Check sheet for the modelled part. Datum: model origin and axes. Units: mm. A direction names the side the tool comes from. Round coordinates to 2 decimals unless told otherwise and drop trailing zeros. Write each loop counter-clockwise with the first axis right and the second up, starting at its lowest first coordinate (ties: lowest second). Pieces come first, ordered by that corner, then holes.
Item 1: Section check A-A, the plane y = -14.5. Record the cut outline in (x, z).
Item 2: Depth check by flat-ended pin: pin 1 (18 mm diameter, centred on y = -20, z = -52.29, fed in from -X); pin 2 (10 mm diameter, centred on y = -25, z = 103, fed in from -X); pin 3 (3 mm diameter, centred on y = -24.5, z = -48.5, fed in from +X). Enter the tip coordinate at first touch or a pass-through.
Item 3: Section check D-D, the plane x = -81. Record the cut outline in (y, z), plus the area to 3 significant figures.
Item 4: Set-up check for faces 1 (the cylindrical face through (73.36, -24.22, -71.32)), 2 (the flat face through (-1, -20, -32.294)), 3 (the flat face through (-12.548, -19.789, 98.794)), 4 (the flat face through (-60, 0, -21)): record each of +Z, -Z, +X, -X, +Y, -Y from which the full face is reachable in a straight line by a thin tool's end or side.
Item 5: Section check C-C, the plane z = -24. Record the cut outline in (x, y).
Item 6: Material ranges on line 1 along Z through (x, y) = (73.5, -20); line 2 along Y through (x, z) = (74, -51); line 3 along Z through (x, y) = (55, -7), recorded low to high.
Item 7: Release check for a two-part mould opening along Z. For faces 5 (the flat face through (86.036, -10, -64)), 6 (the flat face through (-13.932, -0.647, 99.594)), 7 (the flat face through (-38, -20, -72.294)) record: pulls with the +Z half, pulls with the -Z half, needs draft (parallel to the pull), parting line crosses it, or undercut.
Item 8: Section check B-B, the plane x = -21. State how many separate pieces and enclosed holes the cut face has, plus the area to 3 significant figures.
from build123d import *

# Parameters (mm, degrees)
F1_DEPTH = 40
F2_R     = 19.0977324209
F2_R_2   = 15.0689951662
F3_DEPTH = 25
F4_R     = 19.4897068619
F4_R_2   = 15.068995
F5_DEPTH = 25


with BuildPart() as f1:
    # F0 (on Front) → F1 (new body)
    with BuildSketch(Plane.XZ):
        Polygon((61.0357465344, -32.2937653869), (-65.3808493135, -32.2937653869), (4.5902623163, 88.899755018), (-30.0507538351, 108.899755018), (-134.6628816163, -72.2937653869), (61.0357465344, -72.2937653869), align=None)
    extrude(amount=F1_DEPTH)

    # F2 (on face) → F3 (join)
    with BuildSketch(Plane(origin=(39.642288697, 0, 68.6624581515), x_dir=(0.8660254038, 0, -0.5), z_dir=(0.5, 0, 0.8660254038))):
        with Locations((-60.4745937331, -20)):
            Circle(F2_R)
        with Locations((-60.4745937331, -20)):
            Circle(F2_R_2, mode=Mode.SUBTRACT)
    extrude(amount=F3_DEPTH)

    # F4 (on face) → F5 (join)
    with BuildSketch(Plane.YZ.offset(61.0357465344)):
        with Locations((-20, -52.2937653869)):
            Circle(F4_R)
        with Locations((-20, -52.2937653869)):
            Circle(F4_R_2, mode=Mode.SUBTRACT)
    extrude(amount=F5_DEPTH)


solid = f1.part
Values found:
1. outline: (-134.66, -72.29) - (61.04, -72.29) - (61.04, -70.99) - (86.04, -70.99) - (86.04, -66.32) - (61.04, -66.32) - (61.04, -38.26) - (86.04, -38.26) - (86.04, -33.6) - (61.04, -33.6) - (61.04, -32.29) - (-65.38, -32.29) - (4.59, 88.9) - (3.11, 89.76) - (15.61, 111.41) - (11.92, 113.54) - (-0.58, 91.89) - (-24.88, 105.91) - (-12.38, 127.57) - (-16.07, 129.69) - (-28.57, 108.04) - (-30.05, 108.9) - close
2. pin 1: stops at x = -128.31
2. pin 2: stops at x = -36.34
2. pin 3: stops at x = 61.04
3. outline: (-40, -72.29) - (0, -72.29) - (0, 20.65) - (-40, 20.65) - close
3. area: 3,720 mm2
4. face 1: +X
4. face 2: +X, +Y, -Y
4. face 3: none
4. face 4: +Z, -Z, +X, -X, +Y
5. outline: (-106.78, -40) - (-60.59, -40) - (-60.59, 0) - (-106.78, 0) - close
6. line 1: z = -71.78 to -67.36, -37.22 to -32.8
6. line 2: y = -39.45 to -35.01, -4.99 to -0.55
6. line 3: z = -72.29 to -32.29
7. face 5: needs draft
7. face 6: undercut
7. face 7: pulls with the -Z half
8. separate pieces: 2
8. enclosed holes: 1
8. area: 4,230 mm2
